The model under review builds one solid part; all positions refer to its coordinate system, in mm. A direction names the side the tool comes from. Coordinates: 2 decimals unless noted, no trailing zeros. Write each loop counter-clockwise with the first axis right and the second up, starting at its lowest first coordinate (ties: lowest second). Pieces come first, ordered by that corner, then holes. Notation, with made-up numbers: (32, 41) -> (41, 41) arc R19 cw to (41, 60) -> close; hole circle Ø2 at (83, 80.5). An arc over 180 degrees is marked (long way). Write each question's results on one line, items separated by ' | '.
```python
from build123d import *

# Parameters (mm, degrees)
F0_W     = 110.99
F0_H     = 110.99
F0_R     = 1.727
F0_R_2   = 12.5
F1_DEPTH = 6.35
F2_R     = 42.045
F3_DEPTH = 1.6


# Not quite as in the source:
# - a feature names something its author has since deleted; it is built from what else it names


with BuildPart() as f1:
    # F0 (on Front) → F1 (new body)
    with BuildSketch(Plane.XZ):
        Rectangle(F0_W, F0_H)
        with Locations((-46.2755883255, -3.7834937726)):
            Circle(F0_R, mode=Mode.SUBTRACT)
        with Locations((3.7834937726, -46.2755883255)):
            Circle(F0_R, mode=Mode.SUBTRACT)
        with Locations((-3.7834937726, 46.2755883255)):
            Circle(F0_R, mode=Mode.SUBTRACT)
        Circle(F0_R_2, mode=Mode.SUBTRACT)
        with Locations((46.2755883255, 3.7834937726)):
            Circle(F0_R, mode=Mode.SUBTRACT)
    extrude(amount=F1_DEPTH)

    # F2 (on face) → F3 (cut)
    with BuildSketch(Plane.XZ.offset(6.35)):
        Circle(F2_R)
    extrude(amount=-F3_DEPTH, mode=Mode.SUBTRACT)


solid = f1.part
```
Q1. Add section B-B (z = 0). Write out the cut boundary in (x, y) (3 decimals), plus the area to 3 significant figures.
Solution:
outline: (-55.495, -6.35) -> (-42.045, -6.35) -> (-42.045, -4.75) -> (-12.5, -4.75) -> (-12.5, 0) -> (-55.495, 0) -> close; (12.5, -4.75) -> (42.045, -4.75) -> (42.045, -6.35) -> (55.495, -6.35) -> (55.495, 0) -> (12.5, 0) -> close | area: 451 mm²
Q2. For line 1 (Z direction, x = 0, y = -2) (3 decimals); line 2 (Y direction, x = 14, z = 28); line 3 (Z direction, x = -2, y = -4) (3 decimals), list the stretches that pass through material, from the lowest coordinate up. Write a range as from..to.
Solution:
line 1: -55.495..-12.5, 12.5..55.495 | line 2: -4.75..0 | line 3: -55.495..-12.339, 12.339..55.495
Q3. Add section C-C (y = -1.25). Write out the cut boundary in (x, z) (1 decimal), plus the area to 3 significant figures.
Solution:
outline: (-55.5, -55.5) -> (55.5, -55.5) -> (55.5, 55.5) -> (-55.5, 55.5) -> close; hole circle Ø3.5 at (-46.3, -3.8); hole circle Ø25 at (0, 0); hole circle Ø3.5 at (-3.8, 46.3); hole circle Ø3.5 at (3.8, -46.3); hole circle Ø3.5 at (46.3, 3.8) | area: 11,800 mm²
Q4. Clearance check with flat-ended pins moving along their axes: P1, Ø3, axis at x = -46.28, z = -3.78, coming from the -Y side; P2, Ø5, axis at x = 17, z = 35, coming from the -Y side. State where each tip first meets the part, or that it passes through.
Solution:
P1: through | P2: y = -4.75
Q5. Add section D-D (z = 39). Write out the cut boundary in (x, y) (3 decimals), plus the area to 3 significant figures.
Solution:
outline: (-55.495, -6.35) -> (-15.709, -6.35) -> (-15.709, -4.75) -> (15.709, -4.75) -> (15.709, -6.35) -> (55.495, -6.35) -> (55.495, 0) -> (-55.495, 0) -> close | area: 655 mm²
Q6. Add section A-A (x = 0). Write out the cut boundary in (y, z) (3 decimals).
Solution:
outline: (-6.35, -55.495) -> (0, -55.495) -> (0, -12.5) -> (-4.75, -12.5) -> (-4.75, -42.045) -> (-6.35, -42.045) -> close; (-6.35, 42.045) -> (-4.75, 42.045) -> (-4.75, 12.5) -> (0, 12.5) -> (0, 55.495) -> (-6.35, 55.495) -> close
Q7. Machinability: for faces 1 (the flat face through (-10, -4.75, -9)), 2 (the flat face through (-1, 0, 13)), which of the approach directions +Z, -Z, +X, -X, +Y, -Y give a long, thin tool a straight path to every point of the face, cutting with its end or side? Answer none if there is none.
Solution:
face 1: -Y | face 2: +Z, -Z, +X, -X, +Y
